Design review of the part built by this model. Coordinates are the model's own, in mm. Give positions to 0.01 mm unless a question says otherwise; leave off trailing zeros. Order: outer loops, then holes, each group sorted by start corner. A loop starts at its lowest first (then second) coordinate and runs counter-clockwise, first axis right, second up. Notation, with made-up numbers: (38.5, 28.25) -> (50.5, 28.25) arc R21 cw to (50.5, 40.25) -> close; hole circle Ø6 at (33.25, 49). An arc over 180 degrees is marked (long way). One line per item, written item: value. Start each with the question number.
1) Wall thickness on line 1 along X through (y, z) = (1.3, -0.25) (3 decimals); line 2 along Z through (x, y) = (2.75, 1.8); line 3 along Y through (x, z) = (3.75, 5.5) (3 decimals): over which ranges is each line inside the solid? List them lowest first. Write a range as from..to.
2) Consider section B-B (y = 0.2). State the section outline as (x, z) points.
3) For pin 1 (2 mm diameter, centred on x = 9, z = 5.5, fed in from +Y) (3 decimals); pin 2 (0.6 mm diameter, centred on y = 1, z = 3.5, fed in from +X) (3 decimals); pin 3 (0.6 mm diameter, centred on x = 8, y = 1, fed in from -Z), all flat-tipped, find the tip position at first contact; note any pin that passes through.
4) The part is to be moulded in two halves that separate along X. For faces 1 (the face through (6, 0, 1)), 2 (the face through (0, 1, 1)), 3 (the face through (6.4, 0.3, 0)), 4 (the face through (13, 1, 1)), say which applies: released by +X, released by -X, zero draft, split by the parting line, or undercut.
5) Consider section A-A (z = 6.75). State the section outline as (x, y) points (3 decimals).
6) Consider section C-C (x = 2). State the section outline as (y, z) points.
Autodesk Inventor part; units mm, degrees
ref_plane "YZ Plane" through (0, 0, 0) normal (1, 0, 0) x (0, 1, 0)
ref_plane "XZ Plane" through (0, 0, 0) normal (0, 1, 0) x (-1, 0, 0)
ref_plane "XY Plane" through (0, 0, 0) normal (0, 0, 1) x (1, 0, 0)
sketch "Skizze1" plane through (0, 0, 0) normal (0, 0, 1) x (1, 0, 0)
  line L0 (0, 0) -> (13, 0)
  line L1 (13, 0) -> (13, 2)
  line L2 (13, 2) -> (0, 2)
  line L3 (0, 2) -> (0, 0)
  dimension "d0" = 13
  dimension "d1" = 2
extrude "Extrusion1" add sketch "Skizze1" along normal blind 2
sketch "Skizze2" plane through (0, 0, 2) normal (0, 0, 1) x (1, 0, 0)
  line L0 (6.125, 1.375) -> (6.875, 1.375)
  line L1 (6.875, 1.375) -> (6.875, 0.625)
  line L2 (6.875, 0.625) -> (6.125, 0.625)
  line L3 (6.125, 0.625) -> (6.125, 1.375)
  line L4 (13, 2) -> (0, 2) construction
  line L5 (6.5, 2) -> (6.5, 0) construction
  line L6 (0, 0) -> (13, 0) construction
  line L7 (0, 2) -> (0, 0) construction
  line L8 (0, 1) -> (13, 1) construction
  line L9 (13, 0) -> (13, 2) construction
  line L10 (8.875, 1.375) -> (9.625, 1.375)
  line L11 (8.875, 0.625) -> (8.875, 1.375)
  line L12 (9.625, 0.625) -> (8.875, 0.625)
  line L13 (9.625, 1.375) -> (9.625, 0.625)
  line L14 (11.625, 1.375) -> (12.375, 1.375)
  line L15 (11.625, 0.625) -> (11.625, 1.375)
  line L16 (12.375, 0.625) -> (11.625, 0.625)
  line L17 (12.375, 1.375) -> (12.375, 0.625)
  line L18 (3.375, 1.375) -> (4.125, 1.375)
  line L19 (3.375, 0.625) -> (3.375, 1.375)
  line L20 (4.125, 0.625) -> (3.375, 0.625)
  line L21 (4.125, 1.375) -> (4.125, 0.625)
  line L22 (6.125, 1.375) -> (6.875, 1.375)
  line L23 (6.125, 0.625) -> (6.125, 1.375)
  line L24 (6.875, 0.625) -> (6.125, 0.625)
  line L25 (6.875, 1.375) -> (6.875, 0.625)
  line L26 (8.875, 1.375) -> (9.625, 1.375)
  line L27 (8.875, 0.625) -> (8.875, 1.375)
  line L28 (9.625, 0.625) -> (8.875, 0.625)
  line L29 (9.625, 1.375) -> (9.625, 0.625)
  line L30 (0.625, 1.375) -> (1.375, 1.375)
  line L31 (0.625, 0.625) -> (0.625, 1.375)
  line L32 (1.375, 0.625) -> (0.625, 0.625)
  line L33 (1.375, 1.375) -> (1.375, 0.625)
  line L34 (3.375, 1.375) -> (4.125, 1.375)
  line L35 (3.375, 0.625) -> (3.375, 1.375)
  line L36 (4.125, 0.625) -> (3.375, 0.625)
  line L37 (4.125, 1.375) -> (4.125, 0.625)
  line L38 (6.125, 1.375) -> (6.875, 1.375)
  line L39 (6.125, 0.625) -> (6.125, 1.375)
  line L40 (6.875, 0.625) -> (6.125, 0.625)
  line L41 (6.875, 1.375) -> (6.875, 0.625)
  point P0 (6.5, 1.375)
  point P1 (6.125, 1)
  point P2 (9.25, 1.375)
  point P3 (8.875, 1)
  point P4 (12, 1.375)
  point P5 (11.625, 1)
  point P6 (3.75, 1.375)
  point P7 (3.375, 1)
  point P8 (6.5, 1.375)
  point P9 (6.125, 1)
  point P10 (9.25, 1.375)
  point P11 (8.875, 1)
  point P12 (1, 1.375)
  point P13 (0.625, 1)
  point P14 (3.75, 1.375)
  point P15 (3.375, 1)
  point P16 (6.5, 1.375)
  point P17 (6.125, 1)
  dimension "d4" = 0.75
  dimension "d7" = 2.75
  dimension "d10" = 2.75
extrude "Extrusion2" add sketch "Skizze2" along normal blind 6.5
sketch "Skizze3" plane through (0, 0, 0) normal (0, 0, -1) x (-1, 0, 0)
  line L0 (-1.375, 1.375) -> (-0.625, 1.375)
  line L1 (-0.625, 1.375) -> (-0.625, 0.625)
  line L2 (-0.625, 0.625) -> (-1.375, 0.625)
  line L3 (-1.375, 0.625) -> (-1.375, 1.375)
  line L4 (-4.125, 1.375) -> (-3.375, 1.375)
  line L5 (-3.375, 1.375) -> (-3.375, 0.625)
  line L6 (-3.375, 0.625) -> (-4.125, 0.625)
  line L7 (-4.125, 0.625) -> (-4.125, 1.375)
  line L8 (-6.875, 1.375) -> (-6.125, 1.375)
  line L9 (-6.125, 1.375) -> (-6.125, 0.625)
  line L10 (-6.125, 0.625) -> (-6.875, 0.625)
  line L11 (-6.875, 0.625) -> (-6.875, 1.375)
  line L12 (-9.625, 0.625) -> (-9.625, 1.375)
  line L13 (-9.625, 1.375) -> (-8.875, 1.375)
  line L14 (-8.875, 1.375) -> (-8.875, 0.625)
  line L15 (-8.875, 0.625) -> (-9.625, 0.625)
  line L16 (-9.625, 0.625) -> (-9.625, 1.375)
  line L17 (-12.375, 1.375) -> (-11.625, 1.375)
  line L18 (-11.625, 1.375) -> (-11.625, 0.625)
  line L19 (-11.625, 0.625) -> (-12.375, 0.625)
  line L20 (-12.375, 0.625) -> (-12.375, 1.375)
  point P0 (0, 0)
extrude "Extrusion3" add sketch "Skizze3" along normal blind 2
fillet "Rundung1" radius 0.5 4 edges at (0, 0, 1) (0, 2, 1) (13, 0, 1) (13, 2, 1)
properties part number "Pinhead 5"
Checked values:
1. line 1: x = 0.625..1.375, 3.375..4.125, 6.125..6.875, 8.875..9.625, 11.625..12.375
1. line 2: z = 0..2
1. line 3: y = 0.625..1.375
2. outline: (0.1, 0) -> (12.9, 0) -> (12.9, 2) -> (0.1, 2) -> close
3. pin 1: stops at y = 1.375
3. pin 2: stops at x = 12.375
3. pin 3: stops at z = 0
4. face 1: zero draft
4. face 2: released by -X
4. face 3: undercut
4. face 4: released by +X
5. outline: (0.625, 0.625) -> (1.375, 0.625) -> (1.375, 1.375) -> (0.625, 1.375) -> close; (3.375, 0.625) -> (4.125, 0.625) -> (4.125, 1.375) -> (3.375, 1.375) -> close; (6.125, 0.625) -> (6.875, 0.625) -> (6.875, 1.375) -> (6.125, 1.375) -> close; (8.875, 0.625) -> (9.625, 0.625) -> (9.625, 1.375) -> (8.875, 1.375) -> close; (11.625, 0.625) -> (12.375, 0.625) -> (12.375, 1.375) -> (11.625, 1.375) -> close
6. outline: (0, 0) -> (2, 0) -> (2, 2) -> (0, 2) -> close
